Autodesk Inventor part; units mm, degrees
ref_plane "YZ Plane" through (0, 0, 0) normal (1, 0, 0) x (0, 1, 0)
ref_plane "XZ Plane" through (0, 0, 0) normal (0, 1, 0) x (-1, 0, 0)
ref_plane "XY Plane" through (0, 0, 0) normal (0, 0, 1) x (1, 0, 0)
sketch "Sketch1" plane through (0, 0, 0) normal (0, 0, 1) x (1, 0, 0)
  line L0 (0, 6.9282) -> (6, 3.4641)
  line L1 (6, 3.4641) -> (6, -3.4641)
  line L2 (6, -3.4641) -> (0, -6.9282)
  line L3 (0, -6.9282) -> (-6, -3.4641)
  line L4 (-6, -3.4641) -> (-6, 3.4641)
  line L5 (-6, 3.4641) -> (0, 6.9282)
  point P0 (0, 0)
  point P1 (0, 0)
  dimension "d0" = 12
extrude "Extrusion1" add sketch "Sketch1" along normal blind 5.5
sketch "Sketch2" plane through (0, 0, 5.5) normal (0, 0, 1) x (1, 0, 0)
  circle A0 centre (0, 0) radius 4
  dimension "d3" = 8
extrude "Extrusion2" add sketch "Sketch2" along normal blind 4 and the other way blind 14.5
thread "Thread1"
properties part number "hudson-1-46"
Model file for the job. Use its own axes, mm. A direction names the side the tool comes from. Give positions to 0.01 mm unless a question says otherwise; leave off trailing zeros. Order: outer loops, then holes, each group sorted by start corner. A loop starts at its lowest first (then second) coordinate and runs counter-clockwise, first axis right, second up. Notation, with made-up numbers: (-29, 20) -> (13, 20) arc R22 ccw to (13, 52) -> close; hole circle Ø11 at (26, -12.5). An arc over 180 degrees is marked (long way). Use CSV: the item, a comma, the result in double quotes.
1. Band-saw the part on D-D, the plane z = -3. Give the cut face in (x, y).
Outcome:
outline,"circle Ø8 at (0, 0)"
2. Drop flat-ended pins along their axis: pin 1 (2 mm diameter, centred on y = -2.5, z = 7.5, fed in from -X); pin 2 (1.5 mm diameter, centred on y = -1.5, z = 6, fed in from -X); pin 3 (2 mm diameter, centred on y = 3, z = -3.5, fed in from +X); pin 4 (2 mm diameter, centred on x = 2, z = 5.5, fed in from +Y). Give the stop position or say it passes through.
Outcome:
pin 1,"x = -3.71"
pin 2,"x = -6"
pin 3,"x = 3.46"
pin 4,"y = 6.35"
3. Band-saw the part on A-A, the plane y = 0. Give the cut face in (x, z).
Outcome:
outline,"(-6, 0) -> (-4, 0) -> (-4, -9) -> (4, -9) -> (4, 0) -> (6, 0) -> (6, 5.5) -> (4, 5.5) -> (4, 9.5) -> (-4, 9.5) -> (-4, 5.5) -> (-6, 5.5) -> close"
4. Band-saw the part on C-C, the plane z = 1.25. Give the cut face in (x, y), then the cut area to 3 significant figures.
Outcome:
outline,"(-6, -3.46) -> (0, -6.93) -> (6, -3.46) -> (6, 3.46) -> (0, 6.93) -> (-6, 3.46) -> close"
area,"125 mm²"
5. 3-axis set-ups, long thin cutter, end or side, ignore diameter. For faces 4 (the flat face through (-3.042, 5.172, 2.712)), 5 (the flat face through (-3, -3, 5.5)): which of +Z, -Z, +X, -X, +Y, -Y reach the whole face in a straight line?
Outcome:
face 4,"+Z, -Z, -X, +Y"
face 5,"+Z"
6. Band-saw the part on B-B, the plane x = 3.25. Give the cut face in (y, z).
Outcome:
outline,"(-5.05, 0) -> (-2.33, 0) -> (-2.33, -9) -> (2.33, -9) -> (2.33, 0) -> (5.05, 0) -> (5.05, 5.5) -> (2.33, 5.5) -> (2.33, 9.5) -> (-2.33, 9.5) -> (-2.33, 5.5) -> (-5.05, 5.5) -> close"
7. Drill centre lines: line 1 along Z through (x, y) = (3, 5); line 2 along X through (y, z) = (4, 2.5); line 3 along Y through (x, z) = (0.5, -7.25). Where is each one in solid material? Low to high. Write a range as from..to.
Outcome:
line 1,"0..5.5"
line 2,"-5.07..5.07"
line 3,"-3.97..3.97"
8. Mould opens along Z. For faces 1 (the cylindrical face through (-0.867, -3.905, -4.437)), 2 (the flat face through (0, 0, 9.5)), 3 (the flat face through (-3, -3, 0)) say: +Z half, -Z half, draft (parallel to the pull), parting line (faces both ways), or undercut.
Outcome:
face 1,"draft"
face 2,"+Z half"
face 3,"-Z half"
